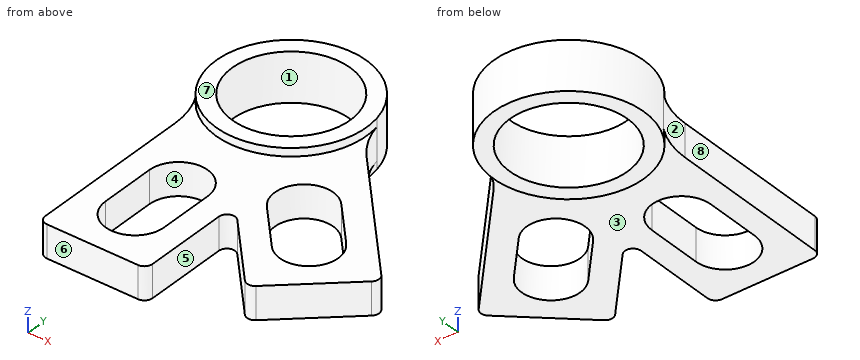
from build123d import *
from build123d.topology import SkipClean

# Parameters (mm, degrees)
SKETCH1_R           = 11.5062
BOSS_EXTRUDE1_DEPTH = 4.7625
CUT_EXTRUDE1_START  = 4.7625
CUT_EXTRUDE1_DEPTH  = 1.5875
CUT_EXTRUDE2_START  = -3.175
CUT_EXTRUDE2_DEPTH  = 1.5875
FILLET1_R           = 1.5875


with BuildPart() as part:
    # Sketch1 → Boss-Extrude1 (new, symmetric)
    # profile 1 of 2: a face of its own
    with BuildSketch(Plane.XY):
        with BuildLine():
            ThreePointArc((-12.661467165, -7.431344606), (5.301915083, -13.690410143), (14.364087476, 3.034901057))
            ThreePointArc((14.364087476, 3.034901057), (15.768494782, -0.923849067), (18.162007104, -4.375683536))
            Line((18.162007104, -4.375683536), (40.915153964, -29.346022579))
            Line((40.915153964, -29.346022579), (25.42603388, -43.459816684))
            Line((25.42603388, -43.459816684), (10.4775, -27.054615176))
            Line((10.4775, -27.054615176), (10.4775, -49.121968099))
            Line((10.4775, -49.121968099), (-10.4775, -49.121968099))
            Line((-10.4775, -49.121968099), (-10.4775, -15.466968099))
            ThreePointArc((-10.4775, -15.466968099), (-11.033218502, -11.303407199), (-12.661467165, -7.431344606))
        make_face()
        with BuildLine():
            ThreePointArc((23.067259929, -16.829899337), (14.993737878, -16.454810433), (14.618648975, -24.528332485))
            Line((14.618648975, -24.528332485), (21.889391392, -32.507576164))
            ThreePointArc((21.889391392, -32.507576164), (29.962913444, -32.882665067), (30.338002347, -24.809143016))
            Line((30.338002347, -24.809143016), (23.067259929, -16.829899337))
        make_face(mode=Mode.SUBTRACT)
        with BuildLine():
            ThreePointArc((5.715, -27.849468099), (0, -22.134468099), (-5.715, -27.849468099))
            Line((-5.715, -27.849468099), (-5.715, -38.644468099))
            ThreePointArc((-5.715, -38.644468099), (0, -44.359468099), (5.715, -38.644468099))
            Line((5.715, -38.644468099), (5.715, -27.849468099))
        make_face(mode=Mode.SUBTRACT)
    # profile 2 of 2: a face of its own
    with BuildSketch(Plane.XY):
        with BuildLine():
            ThreePointArc((14.364087476, 3.034901057), (-5.301915083, 13.690410143), (-12.661467165, -7.431344606))
            ThreePointArc((-12.661467165, -7.431344606), (5.301915083, -13.690410143), (14.364087476, 3.034901057))
        make_face()
        with Locations(Location((0, 0, 0), (0, 0, 180))):
            Circle(SKETCH1_R, mode=Mode.SUBTRACT)
    extrude(amount=BOSS_EXTRUDE1_DEPTH, both=True)

    # Sketch3 → Cut-Extrude1 (cut)
    with SkipClean():  # the faces are left unmerged after this step: merging them gives an invalid solid
        with BuildSketch(Plane.XY.offset(CUT_EXTRUDE1_START)):
            with BuildLine():
                ThreePointArc((-12.661467165, -7.431344606), (5.301915083, -13.690410143), (14.364087476, 3.034901057))
                ThreePointArc((14.364087476, 3.034901057), (15.768494782, -0.923849067), (18.162007104, -4.375683536))
                Line((18.162007104, -4.375683536), (40.915153964, -29.346022579))
                Line((40.915153964, -29.346022579), (25.42603388, -43.459816684))
                Line((25.42603388, -43.459816684), (10.4775, -27.054615176))
                Line((10.4775, -27.054615176), (10.4775, -49.121968099))
                Line((10.4775, -49.121968099), (-10.4775, -49.121968099))
                Line((-10.4775, -49.121968099), (-10.4775, -15.466968099))
                ThreePointArc((-10.4775, -15.466968099), (-11.033218502, -11.303407199), (-12.661467165, -7.431344606))
            make_face()
            with BuildLine():
                ThreePointArc((23.067259929, -16.829899337), (14.993737878, -16.454810433), (14.618648975, -24.528332485))
                Line((14.618648975, -24.528332485), (21.889391392, -32.507576164))
                ThreePointArc((21.889391392, -32.507576164), (29.962913444, -32.882665067), (30.338002347, -24.809143016))
                Line((30.338002347, -24.809143016), (23.067259929, -16.829899337))
            make_face(mode=Mode.SUBTRACT)
            with BuildLine():
                ThreePointArc((5.715, -27.849468099), (0, -22.134468099), (-5.715, -27.849468099))
                Line((-5.715, -27.849468099), (-5.715, -38.644468099))
                ThreePointArc((-5.715, -38.644468099), (0, -44.359468099), (5.715, -38.644468099))
                Line((5.715, -38.644468099), (5.715, -27.849468099))
            make_face(mode=Mode.SUBTRACT)
        extrude(amount=-CUT_EXTRUDE1_DEPTH, mode=Mode.SUBTRACT)

    # Sketch3<11> → Cut-Extrude2 (cut)
    with SkipClean():  # the faces are left unmerged after this step: merging them gives an invalid solid
        with BuildSketch(Plane.XY.offset(CUT_EXTRUDE2_START)):
            with BuildLine():
                ThreePointArc((-12.661467165, -7.431344606), (5.301915083, -13.690410143), (14.364087476, 3.034901057))
                ThreePointArc((14.364087476, 3.034901057), (15.768494782, -0.923849067), (18.162007104, -4.375683536))
                Line((18.162007104, -4.375683536), (40.915153964, -29.346022579))
                Line((40.915153964, -29.346022579), (25.42603388, -43.459816684))
                Line((25.42603388, -43.459816684), (10.4775, -27.054615176))
                Line((10.4775, -27.054615176), (10.4775, -49.121968099))
                Line((10.4775, -49.121968099), (-10.4775, -49.121968099))
                Line((-10.4775, -49.121968099), (-10.4775, -15.466968099))
                ThreePointArc((-10.4775, -15.466968099), (-11.033218502, -11.303407199), (-12.661467165, -7.431344606))
            make_face()
            with BuildLine():
                ThreePointArc((23.067259929, -16.829899337), (14.993737878, -16.454810433), (14.618648975, -24.528332485))
                Line((14.618648975, -24.528332485), (21.889391392, -32.507576164))
                ThreePointArc((21.889391392, -32.507576164), (29.962913444, -32.882665067), (30.338002347, -24.809143016))
                Line((30.338002347, -24.809143016), (23.067259929, -16.829899337))
            make_face(mode=Mode.SUBTRACT)
            with BuildLine():
                ThreePointArc((5.715, -27.849468099), (0, -22.134468099), (-5.715, -27.849468099))
                Line((-5.715, -27.849468099), (-5.715, -38.644468099))
                ThreePointArc((-5.715, -38.644468099), (0, -44.359468099), (5.715, -38.644468099))
                Line((5.715, -38.644468099), (5.715, -27.849468099))
            make_face(mode=Mode.SUBTRACT)
        extrude(amount=-CUT_EXTRUDE2_DEPTH, mode=Mode.SUBTRACT)

    # Fillet1
    fillet1_edges = [part.edges().sort_by_distance(p)[0] for p in [
        (40.915153964, -29.346022579, 0),
        (25.42603388, -43.459816684, 0),
        (10.4775, -27.054615176, 0),
        (10.4775, -49.121968099, 0),
        (-10.4775, -49.121968099, 0),
    ]]
    fillet(fillet1_edges, radius=FILLET1_R)


solid = part.part
The listing builds one solid part. Answer for the finished solid, in the listing's coordinates (mm). Face numbers are marked on the shaded views. A direction names the side the tool comes from. Give positions to 0.01 mm unless a question says otherwise; leave off trailing zeros. Order: outer loops, then holes, each group sorted by start corner. A loop starts at its lowest first (then second) coordinate and runs counter-clockwise, first axis right, second up. Notation, with made-up numbers: (71, 4.25) - (111, 4.25) arc R19 cw to (111, 10.25) - close; hole circle Ø10 at (53.25, 27). An arc over 180 degrees is marked (long way). One line per item, written item: value. Start each with the question number.
1) A cutting plane is placed at A-A on x = 0. Give the vertices of the cut face in (y, z) (1 decimal), then the cut area to 3 significant figures.
2) A cutting plane is placed at C-C on z = -1.25. State how many separate pieces and enclosed holes the cut face has, then the cut area to 3 significant figures.
3) A cutting plane is placed at D-D on x = 7. Give the vertices of the cut face in (y, z) (1 decimal), then the cut area to 3 significant figures.
4) The mould has two halves that part along Y. Classify the marked faces 1, 2 and 3: released by +Y, released by -Y, zero draft, split by the parting line, or undercut.
5) A tool of negligible diameter and unlimited length cuts with its end or side. For the marked faces 4, 5, 6, 7 and 8, from which of +Z, -Z, +X, -X, +Y, -Y can it reach the whole face along a straight path? Write none if from no direction.
6) Find the intervals of material crossed by L1, parallel to Y at x = 0, z = 2.25; L2, parallel to X at y = 5, z = -1.75; L3, parallel to X at y = 9, z = -3.5, in increasing order.
7) A cutting plane is placed at B-B on y = -10.5. Give the vertices of the cut face in (x, z) (1 decimal), then the cut area to 3 significant figures.
8) Given pin 1 Ø1 at (x, y) = (10.5, -20.5) entering from +Z (3 decimals); pin 2 Ø15.5 at (x, y) = (9.5, -25.5) entering from -Z (3 decimals); pin 3 Ø3 at (y, z) = (-39.5, 3) entering from +X, each flat-ended and moving along its own axis, determine where each tip first touches the part or whether it passes through.
Answer sheet:
1. outline: (-49.1, -3.2) - (-44.4, -3.2) - (-44.4, 3.2) - (-49.1, 3.2) - close; (-22.1, -3.2) - (-14.7, -3.2) - (-14.7, -4.8) - (-11.5, -4.8) - (-11.5, 4.8) - (-14.7, 4.8) - (-14.7, 3.2) - (-22.1, 3.2) - close; (11.5, -4.8) - (14.7, -4.8) - (14.7, 4.8) - (11.5, 4.8) - close
1. area: 138 mm2
2. separate pieces: 1
2. enclosed holes: 3
2. area: 1,230 mm2
3. outline: (-49.1, -3.2) - (-12.9, -3.2) - (-12.9, -4.8) - (-9.1, -4.8) - (-9.1, 4.8) - (-12.9, 4.8) - (-12.9, 3.2) - (-49.1, 3.2) - close; (9.1, -4.8) - (12.9, -4.8) - (12.9, 4.8) - (9.1, 4.8) - close
3. area: 302 mm2
4. face 1: undercut
4. face 2: released by -Y
4. face 3: zero draft
5. face 4: +Z, -Z
5. face 5: +Z, -Z, -Y
5. face 6: +Z, -Z, +X, -X, -Y
5. face 7: +Z, +X, -X, +Y, -Y
5. face 8: +Z, -Z, -X, -Y
6. L1: y = -49.12 to -44.36, -22.13 to -11.51, 11.51 to 14.68
6. L2: x = -13.8 to -10.36, 10.36 to 13.8
6. L3: x = -11.6 to -7.17, 7.17 to 11.6
7. outline: (-11.3, -3.2) - (-10.3, -3.2) - (-10.3, -4.8) - (-4.7, -4.8) - (-4.7, 4.8) - (-10.3, 4.8) - (-10.3, 3.2) - (-11.3, 3.2) - close; (4.7, -4.8) - (10.3, -4.8) - (10.3, -3.2) - (23.7, -3.2) - (23.7, 3.2) - (10.3, 3.2) - (10.3, 4.8) - (4.7, 4.8) - close
7. area: 198 mm2
8. pin 1: stops at z = 3.175
8. pin 2: stops at z = -3.175
8. pin 3: stops at x = 31.42
